```python
from build123d import *

# Parameters (mm, degrees)
BOSS_EXTRUDE1_DEPTH = 5
SKETCH4_W           = 5
SKETCH4_H           = 30
BOSS_EXTRUDE4_DEPTH = 35
SKETCH5_R           = 3
CUT_EXTRUDE2_DEPTH  = 40
CUT_EXTRUDE3_DEPTH  = 10
SKETCH7_R           = 1
SKETCH7_R_2         = 1.000000019
CUT_EXTRUDE4_DEPTH  = 10
FILLET2_R           = 3
FILLET3_R           = 3
FILLET5_R           = 3
FILLET6_R           = 3
SKETCH8_R           = 1.45
CUT_EXTRUDE6_DEPTH  = 4


with BuildPart() as part:
    # Sketch1 → Boss-Extrude1 (new body)
    with BuildSketch(Plane.XY):
        with BuildLine():
            Line((5, 0), (36.35, 0))
            Line((36.35, 0), (36.35, 15))
            Line((36.35, 15), (-36.35, 15))
            Line((-36.35, 15), (-36.35, 0))
            Line((-36.35, 0), (-5, 0))
            ThreePointArc((-5, 0), (0, 5), (5, 0))
        make_face()
        with BuildLine():
            ThreePointArc((-5, 0), (0, -5), (5, 0))
            Line((5, 0), (0, 0))
            Line((0, 0), (-5, 0))
        make_face()
        with BuildLine():
            Line((0, 0), (5, 0))
            ThreePointArc((5, 0), (0, 5), (-5, 0))
            Line((-5, 0), (0, 0))
        make_face()
        with BuildLine():
            Line((-36.35, -15), (36.35, -15))
            Line((36.35, -15), (36.35, 0))
            Line((36.35, 0), (5, 0))
            ThreePointArc((5, 0), (0, -5), (-5, 0))
            Line((-5, 0), (-36.35, 0))
            Line((-36.35, 0), (-36.35, -15))
        make_face()
    extrude(amount=BOSS_EXTRUDE1_DEPTH)

    # Sketch4 → Boss-Extrude4 (add)
    with BuildSketch(Plane(origin=(0, 0, 0), x_dir=(-1, 0, 0), z_dir=(0, 0, -1))):
        with Locations((-33.85, 0)):
            Rectangle(SKETCH4_W, SKETCH4_H)
    boss_extrude4 = extrude(amount=BOSS_EXTRUDE4_DEPTH)

    # Sketch5 → Cut-Extrude2 (cut)
    with BuildSketch(Plane(origin=(36.35, 0, 0), x_dir=(0, 0, -1), z_dir=(1, 0, 0))):
        with Locations(Location((20, 0, 0), (0, 0, 90))):
            Circle(SKETCH5_R)
    cut_extrude2 = extrude(amount=-CUT_EXTRUDE2_DEPTH, mode=Mode.SUBTRACT)

    # Sketch6 → Cut-Extrude3 (cut)
    with BuildSketch(Plane.ZY.offset(-31.35)):
        with BuildLine():
            ThreePointArc((-35, 0), (-30.606601718, 10.606601718), (-20, 15))
            Line((-20, 15), (-35, 15))
            Line((-35, 15), (-35, 0))
        make_face()
        with BuildLine():
            ThreePointArc((-20, -15), (-30.606601718, -10.606601718), (-35, 0))
            Line((-35, 0), (-35, -15))
            Line((-35, -15), (-20, -15))
        make_face()
    cut_extrude3 = extrude(amount=-CUT_EXTRUDE3_DEPTH, mode=Mode.SUBTRACT)

    # Sketch7 → Cut-Extrude4 (cut)
    with BuildSketch(Plane.ZY.offset(-31.35)):
        with Locations((-28.485281374, 8.485281374)):
            Circle(SKETCH7_R)
        with Locations((-11.514718626, 8.485281374)):
            Circle(SKETCH7_R)
        with Locations((-8, 0)):
            Circle(SKETCH7_R)
        with Locations((-32, -2e-08)):
            Circle(SKETCH7_R_2)
        with Locations((-11.514718626, -8.485281374)):
            Circle(SKETCH7_R)
        with Locations((-20, 12)):
            Circle(SKETCH7_R)
        with Locations((-28.485281374, -8.485281374)):
            Circle(SKETCH7_R)
        with Locations((-20, -12)):
            Circle(SKETCH7_R)
    cut_extrude4 = extrude(amount=-CUT_EXTRUDE4_DEPTH, mode=Mode.SUBTRACT)

    # Fillet2
    fillet2_edges = [part.edges().sort_by_distance(p)[0] for p in [
        (36.35, 0, 5),
    ]]
    fillet(fillet2_edges, radius=FILLET2_R)

    # Fillet3
    fillet3_edges = [part.edges().sort_by_distance(p)[0] for p in [
        (31.35, 0, 0),
    ]]
    fillet(fillet3_edges, radius=FILLET3_R)

    # Mirror2: Boss-Extrude4, Cut-Extrude2, Cut-Extrude3, Cut-Extrude4 across plane
    add(boss_extrude4.mirror(Plane(origin=(0, 0, 0), x_dir=(0, 0, 1), z_dir=(1, 0, 0))))
    add(cut_extrude2.mirror(Plane(origin=(0, 0, 0), x_dir=(0, 0, 1), z_dir=(1, 0, 0))), mode=Mode.SUBTRACT)
    add(cut_extrude3.mirror(Plane(origin=(0, 0, 0), x_dir=(0, 0, 1), z_dir=(1, 0, 0))), mode=Mode.SUBTRACT)
    add(cut_extrude4.mirror(Plane(origin=(0, 0, 0), x_dir=(0, 0, 1), z_dir=(1, 0, 0))), mode=Mode.SUBTRACT)

    # Fillet5
    fillet5_edges = [part.edges().sort_by_distance(p)[0] for p in [
        (-36.35, 0, 5),
    ]]
    fillet(fillet5_edges, radius=FILLET5_R)

    # Fillet6
    fillet6_edges = [part.edges().sort_by_distance(p)[0] for p in [
        (-31.35, 0, 0),
    ]]
    fillet(fillet6_edges, radius=FILLET6_R)

    # Sketch8 → Cut-Extrude6 (cut)
    with BuildSketch(Plane.XY.offset(5)):
        with Locations((-18.1, 10)):
            Circle(SKETCH8_R)
        with Locations((18.1, 10)):
            Circle(SKETCH8_R)
        with Locations((18.1, -10)):
            Circle(SKETCH8_R)
        with Locations((-18.1, -10)):
            Circle(SKETCH8_R)
    extrude(amount=-CUT_EXTRUDE6_DEPTH, mode=Mode.SUBTRACT)


solid = part.part
```
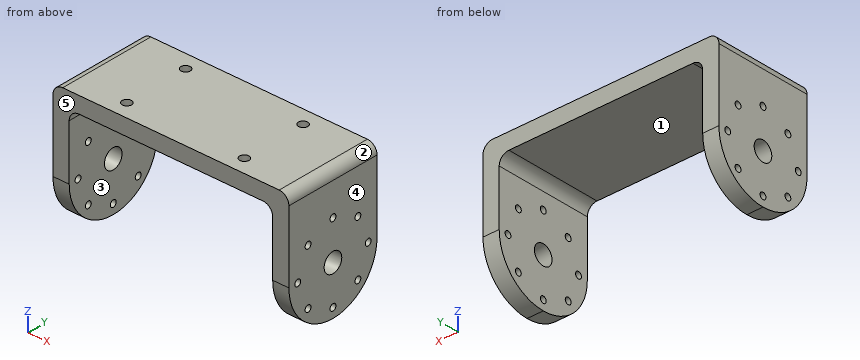
CAD build for the part. Positions are in the model's coordinates, mm. Face numbers are marked on the shaded views. A direction names the side the tool comes from. Round coordinates to 2 decimals unless told otherwise and drop trailing zeros. Loops run counter-clockwise (first coordinate to the right, second up) from the corner with the lowest first, then second, coordinate; pieces in that order, holes last. Notation, with made-up numbers: (-11.5, 37) - (16.5, 37) arc R29 cw to (16.5, 57) - close; hole circle Ø4 at (35, 78.25). An arc over 180 degrees is marked (long way). Return JSON: item names as keys, results as strings. Group by question number.
Q1. Tool access for the marked faces 1 and 2: list every direction of +Z, -Z, +X, -X, +Y, -Y with a clear straight run to the whole face (end or side of a thin tool).
Q2. Flat gauge pins, fed straight in: pin 1 Ø6 at (x, y) = (-20.5, 5) entering from -Z; pin 2 Ø1.8 at (y, z) = (0, -32) entering from +X (1 decimal); pin 3 Ø1.4 at (x, y) = (18, -9.5) entering from +Z; pin 4 Ø3 at (y, z) = (8.49, -11.51) entering from +X. Where does each tip first touch, or does it go through?
Q3. Drill centre lines: line 1 along Y through (x, z) = (-18.1, 2.65); line 2 along Y through (x, z) = (31.5, -11.5); line 3 along X through (y, z) = (8.75, -14.5). Where is each one in solid material? Low to high. Write a range as [from, to].
Q4. Band-saw the part on B-B on x = 18.1. Give the cut face in (y, z).
Q5. Band-saw the part on D-D on y = 6.75. Give the cut face in (x, z).
Q6. Band-saw the part on C-C on z = -8. Give the cut face in (x, y).
Q7. Band-saw the part on A-A on z = -32. Give the cut face in (x, y), plus the area to 3 significant figures.
Q8. Two-plate mould, pull along X, no slides. Class the marked faces 3, 4 and 5: +X half, -X half, draft (parallel to the pull), parting line (faces both ways), or undercut.
Solutions:
{
 "1": {"face 1": "-Z, +Y, -Y", "face 2": "+Z, +X, +Y, -Y"},
 "2": {"pin 1": "stops at z = 0", "pin 2": "passes through", "pin 3": "stops at z = 1", "pin 4": "stops at x = 36.35"},
 "3": {"line 1": "y = [-15, -11.45], [-8.55, 8.55], [11.45, 15]", "line 2": "y = [-15, -9.49], [-7.49, 7.49], [9.49, 15]", "line 3": "x = [-36.35, -31.35], [31.35, 36.35]"},
 "4": {"outline": "(-15, 0) - (15, 0) - (15, 5) - (11.45, 5) - (11.45, 1) - (8.55, 1) - (8.55, 5) - (-8.55, 5) - (-8.55, 1) - (-11.45, 1) - (-11.45, 5) - (-15, 5) - close"},
 "5": {"outline": "(-36.35, -33.4) - (-31.35, -33.4) - (-31.35, -3) arc R3 cw to (-28.35, 0) - (28.35, 0) arc R3 cw to (31.35, -3) - (31.35, -33.4) - (36.35, -33.4) - (36.35, 2) arc R3 ccw to (33.35, 5) - (-33.35, 5) arc R3 ccw to (-36.35, 2) - close"},
 "6": {"outline": "(-36.35, -15) - (-31.35, -15) - (-31.35, -1) - (-36.35, -1) - close; (-36.35, 1) - (-31.35, 1) - (-31.35, 15) - (-36.35, 15) - close; (31.35, -15) - (36.35, -15) - (36.35, -1) - (31.35, -1) - close; (31.35, 1) - (36.35, 1) - (36.35, 15) - (31.35, 15) - close"},
 "7": {"outline": "(-36.35, -9) - (-31.35, -9) - (-31.35, -1) - (-36.35, -1) - close; (-36.35, 1) - (-31.35, 1) - (-31.35, 9) - (-36.35, 9) - close; (31.35, -9) - (36.35, -9) - (36.35, -1) - (31.35, -1) - close; (31.35, 1) - (36.35, 1) - (36.35, 9) - (31.35, 9) - close", "area": "160 mm^2"},
 "8": {"face 3": "undercut", "face 4": "+X half", "face 5": "draft"}
}
